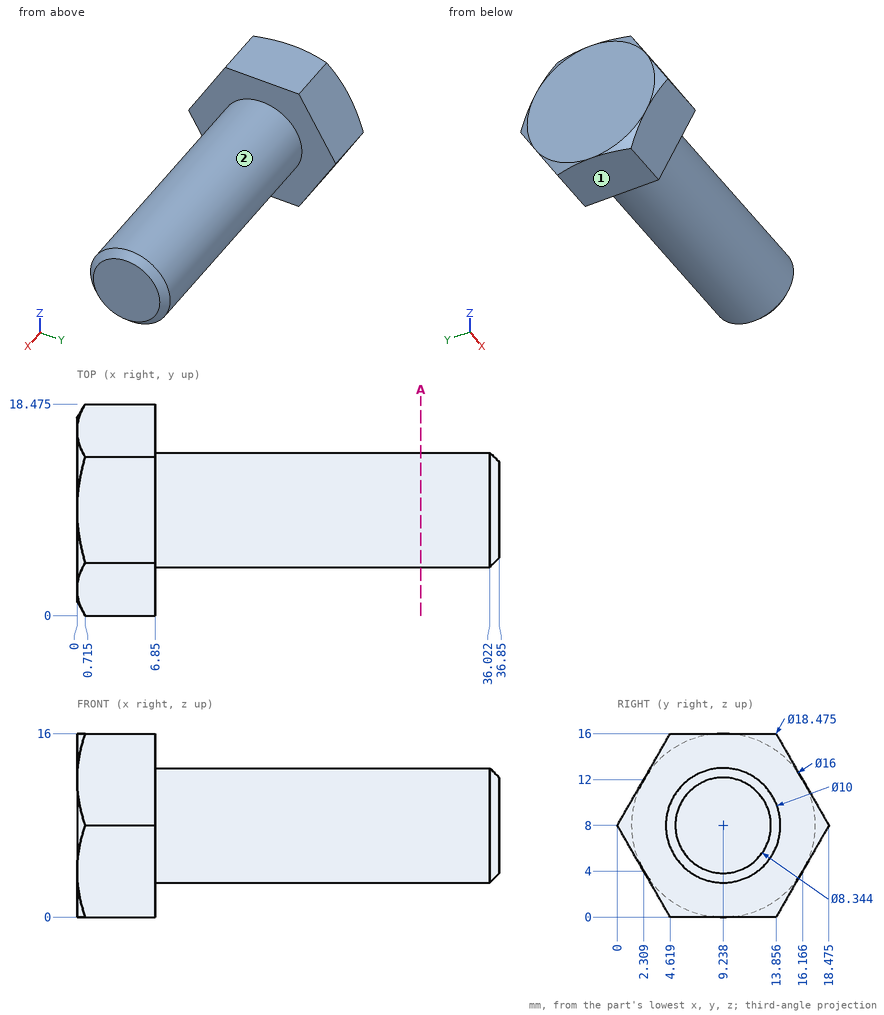
Part print with two shaded views. Sizes in mm from the minimum x, y, z corner. A direction names the side the tool comes from. Round coordinates to 2 decimals unless told otherwise and drop trailing zeros. Order: outer loops, then holes, each group sorted by start corner. A loop starts at its lowest first (then second) coordinate and runs counter-clockwise, first axis right, second up. Notation, with made-up numbers: M 42.5,48.5 L 69.5,48.5 A10 cw 69.5,60.5 Z; hole C 0,26 d6. An arc over 180 degrees is marked long. Put each result on its own line as item: value. Start each with the question number.
1. Slice it at A-A on x = 30. List the corners of the cut face in (y, z).
2. Drop flat-ended pins along their axis: pin 1 (3 mm diameter, centred on x = 21.5, y = 13.5, fed in from +Z); pin 2 (8 mm diameter, centred on x = 31, z = 9.5, fed in from +Y); pin 3 (10 mm diameter, centred on x = 25.5, y = 4.5, fed in from +Z). Give the stop position or say it passes through.
3. Drill centre lines: probe 1 along X at (y, z) = (16.5, 9.25); probe 2 along Y at (x, z) = (3, 12) (1 decimal); probe 3 along Y at (x, z) = (4.5, 2.75) (1 decimal). Where is each one in solid material? Low to high. Write a range as [from, to].
4. Tool access for the marked faces 1 and 2: list every direction of +Z, -Z, +X, -X, +Y, -Y with a clear straight run to the whole face (end or side of a thin tool).
Findings:
1. outline: C 9.24,8 d10
2. pin 1: z = 12.17
2. pin 2: y = 14.24
2. pin 3: z = 13
3. probe 1: [0, 6.85]
3. probe 2: [2.3, 16.2]
3. probe 3: [3, 15.4]
4. face 1: -Z, +X, -X, +Y, -Y
4. face 2: +X
